For this review, take the finished solid that the model builds, in its own axes (mm). Round coordinates to 2 decimals unless told otherwise and drop trailing zeros. Order: outer loops, then holes, each group sorted by start corner. A loop starts at its lowest first (then second) coordinate and runs counter-clockwise, first axis right, second up. Notation, with made-up numbers: (26, -1.5) -> (56, -1.5) arc R33 cw to (56, 32.5) -> close; hole circle Ø7 at (10.25, 6.5). An arc over 180 degrees is marked (long way). Use a Markdown table: item, result. Add a question column.
1) Consider section D-D (z = 1). Give the number of separate pieces and of enclosed holes in the cut face, plus the area to 3 significant figures.
2) Consider section C-C (x = -10). State the section outline as (y, z) points.
3) Clearance check with flat-ended pins moving along their axes: P1, Ø2, axis at x = -4, z = 3, coming from the +Y side; P2, Ø6, axis at x = -12.5, y = -0.5, coming from the -Z side; P3, Ø2, axis at x = 10, z = 0.5, coming from the +Y side; P4, Ø1, axis at y = -2.5, z = 2, coming from the +X side. State where each tip first meets the part, or that it passes through.
4) Draft analysis for pull direction X (two halves, no side actions). For faces 1 (the face through (-0.193, -19.374, 1.972)), 2 (the face through (6.763, 13.463, 1.972)), 3 (the face through (-19.374, 0.193, 1.972)), state which applies: pulls with the +X half, pulls with the -X half, needs draft (parallel to the pull), parting line crosses it, or undercut.
5) Wall thickness on line 1 along Y through (x, z) = (0, 2.2) (3 decimals); line 2 along X through (y, z) = (2, 1.9); line 3 along X through (y, z) = (0.5, 3.85): over which ranges is each line inside the solid? List them lowest first. Write a range as [from, to].
6) Consider section A-A (x = 0). State the section outline as (y, z) points (3 decimals).
```python
from build123d import *

# Parameters (mm, degrees)
SKETCH1_R           = 19.375
SKETCH1_R_2         = 9
BOSS_EXTRUDE1_DEPTH = 4
CUT_EXTRUDE1_DEPTH  = 4
FILLET1_R           = 0.5
CUT_EXTRUDE2_DEPTH  = 10


with BuildPart() as part:
    # Sketch1 → Boss-Extrude1 (new body)
    with BuildSketch(Plane.XY):
        Circle(SKETCH1_R)
        Circle(SKETCH1_R_2, mode=Mode.SUBTRACT)
        with BuildLine():
            Line((6.689691504, 12.241024694), (6.226047976, 11.350373764))
            ThreePointArc((6.226047976, 11.350373764), (5.41320923, 10.635157913), (4.330662681, 10.653420143))
            ThreePointArc((4.330662681, 10.653420143), (0, 11.5), (-4.330662681, 10.653420143))
            ThreePointArc((-4.330662681, 10.653420143), (-5.41320923, 10.635157913), (-6.226047976, 11.350373764))
            Line((-6.226047976, 11.350373764), (-6.689691504, 12.241024694))
            ThreePointArc((-6.689691504, 12.241024694), (-6.768746058, 13.446590252), (-5.933372603, 14.319395572))
            ThreePointArc((-5.933372603, 14.319395572), (0, 15.5), (5.933372603, 14.319395572))
            ThreePointArc((5.933372603, 14.319395572), (6.768746058, 13.446590252), (6.689691504, 12.241024694))
        make_face(mode=Mode.SUBTRACT)
        with BuildLine():
            Line((12.241024694, 6.689691504), (11.350373764, 6.226047976))
            ThreePointArc((11.350373764, 6.226047976), (10.635157913, 5.41320923), (10.653420143, 4.330662681))
            ThreePointArc((10.653420143, 4.330662681), (11.5, 0), (10.653420143, -4.330662681))
            ThreePointArc((10.653420143, -4.330662681), (10.635157913, -5.41320923), (11.350373764, -6.226047976))
            Line((11.350373764, -6.226047976), (12.241024694, -6.689691504))
            ThreePointArc((12.241024694, -6.689691504), (13.446590252, -6.768746058), (14.319395572, -5.933372603))
            ThreePointArc((14.319395572, -5.933372603), (15.5, 0), (14.319395572, 5.933372603))
            ThreePointArc((14.319395572, 5.933372603), (13.446590252, 6.768746058), (12.241024694, 6.689691504))
        make_face(mode=Mode.SUBTRACT)
        with BuildLine():
            Line((6.689691504, -12.241024694), (6.226047976, -11.350373764))
            ThreePointArc((6.226047976, -11.350373764), (5.41320923, -10.635157913), (4.330662681, -10.653420143))
            ThreePointArc((4.330662681, -10.653420143), (0, -11.5), (-4.330662681, -10.653420143))
            ThreePointArc((-4.330662681, -10.653420143), (-5.41320923, -10.635157913), (-6.226047976, -11.350373764))
            Line((-6.226047976, -11.350373764), (-6.689691504, -12.241024694))
            ThreePointArc((-6.689691504, -12.241024694), (-6.768746058, -13.446590252), (-5.933372603, -14.319395572))
            ThreePointArc((-5.933372603, -14.319395572), (0, -15.5), (5.933372603, -14.319395572))
            ThreePointArc((5.933372603, -14.319395572), (6.768746058, -13.446590252), (6.689691504, -12.241024694))
        make_face(mode=Mode.SUBTRACT)
        with BuildLine():
            Line((-12.241024694, -6.689691504), (-11.350373764, -6.226047976))
            ThreePointArc((-11.350373764, -6.226047976), (-10.635157913, -5.41320923), (-10.653420143, -4.330662681))
            ThreePointArc((-10.653420143, -4.330662681), (-11.5, 0), (-10.653420143, 4.330662681))
            ThreePointArc((-10.653420143, 4.330662681), (-10.635157913, 5.41320923), (-11.350373764, 6.226047976))
            Line((-11.350373764, 6.226047976), (-12.241024694, 6.689691504))
            ThreePointArc((-12.241024694, 6.689691504), (-13.446590252, 6.768746058), (-14.319395572, 5.933372603))
            ThreePointArc((-14.319395572, 5.933372603), (-15.5, 0), (-14.319395572, -5.933372603))
            ThreePointArc((-14.319395572, -5.933372603), (-13.446590252, -6.768746058), (-12.241024694, -6.689691504))
        make_face(mode=Mode.SUBTRACT)
    extrude(amount=BOSS_EXTRUDE1_DEPTH)

    # Sketch2 → Cut-Extrude1 (cut)
    with BuildSketch(Plane(origin=(0, 0, 0), x_dir=(-1, 0, 0), z_dir=(0, 0, -1))):
        Polygon((10.65368142, -8.367490994), (8.367490994, -10.65368142), (9.204294768, -13.776675621), (12.327288968, -14.613479395), (14.613479395, -12.327288968), (13.776675621, -9.204294768), align=None)
        Polygon((13.776675621, 9.204294768), (14.613479395, 12.327288968), (12.327288968, 14.613479395), (9.204294768, 13.776675621), (8.367490994, 10.65368142), (10.65368142, 8.367490994), align=None)
        Polygon((-8.367490994, -10.65368142), (-10.65368142, -8.367490994), (-13.776675621, -9.204294768), (-14.613479395, -12.327288968), (-12.327288968, -14.613479395), (-9.204294768, -13.776675621), align=None)
        Polygon((-10.65368142, 8.367490994), (-8.367490994, 10.65368142), (-9.204294768, 13.776675621), (-12.327288968, 14.613479395), (-14.613479395, 12.327288968), (-13.776675621, 9.204294768), align=None)
    extrude(amount=-CUT_EXTRUDE1_DEPTH, mode=Mode.SUBTRACT)

    # Fillet1
    fillet1_edges = [part.edges().sort_by_distance(p)[0] for p in [
        (-9, 0, 0),
        (-9, 0, 4),
    ]]
    fillet(fillet1_edges, radius=FILLET1_R)

    # Sketch3 → Cut-Extrude2 (cut)
    with BuildSketch(Plane.XY.offset(4)):
        Polygon((-13.776675621, 9.204294768), (-15.450283169, 15.450283169), (-9.204294768, 13.776675621), align=None)
        Polygon((9.204294768, 13.776675621), (15.450283169, 15.450283169), (13.776675621, 9.204294768), align=None)
        Polygon((13.776675621, -9.204294768), (15.450283169, -15.450283169), (9.204294768, -13.776675621), align=None)
        Polygon((-9.204294768, -13.776675621), (-15.450283169, -15.450283169), (-13.776675621, -9.204294768), align=None)
    extrude(amount=-CUT_EXTRUDE2_DEPTH, mode=Mode.SUBTRACT)


solid = part.part
```
Results list:
| question | item | result |
|---|---|---|
| 1 | separate pieces | 1 |
| 1 | enclosed holes | 5 |
| 1 | area | 604 mm2 |
| 2 | outline | (-16.59, 0) -> (-13.99, 0) -> (-13.99, 4) -> (-16.59, 4) -> close; (-9.02, 0) -> (9.02, 0) -> (9.02, 4) -> (-9.02, 4) -> close; (13.99, 0) -> (16.59, 0) -> (16.59, 4) -> (13.99, 4) -> close |
| 3 | P1 | y = 19.14 |
| 3 | P2 | z = 0 |
| 3 | P3 | y = 17.16 |
| 3 | P4 | x = 19.27 |
| 4 | face 1 | parting line crosses it |
| 4 | face 2 | undercut |
| 4 | face 3 | pulls with the -X half |
| 5 | line 1 | [-19.375, -15.5], [-11.5, -9], [9, 11.5], [15.5, 19.375] |
| 5 | line 2 | [-19.27, -15.37], [-11.32, -8.77], [8.77, 11.32], [15.37, 19.27] |
| 5 | line 3 | [-19.37, -15.49], [-11.49, -9.13], [9.13, 11.49], [15.49, 19.37] |
| 6 | outline | (-19.375, 0) -> (-15.5, 0) -> (-15.5, 4) -> (-19.375, 4) -> close; (-11.5, 0) -> (-9.5, 0) arc R0.5 ccw to (-9, 0.5) -> (-9, 3.5) arc R0.5 ccw to (-9.5, 4) -> (-11.5, 4) -> close; (9, 0.5) arc R0.5 ccw to (9.5, 0) -> (11.5, 0) -> (11.5, 4) -> (9.5, 4) arc R0.5 ccw to (9, 3.5) -> close; (15.5, 0) -> (19.375, 0) -> (19.375, 4) -> (15.5, 4) -> close |
